Geometry: final body of the model. Coordinates: model frame, mm. A direction names the side the tool comes from. Round coordinates to 2 decimals unless told otherwise and drop trailing zeros. Loops run counter-clockwise (first coordinate to the right, second up) from the corner with the lowest first, then second, coordinate; pieces in that order, holes last. Notation, with made-up numbers: (-15.5, 80) - (21.5, 80) arc R21 ccw to (21.5, 93) - close; hole circle Ø5 at (-27, 3.5). An arc over 180 degrees is marked (long way). Use CSV: the item, a comma, the result in double quotes.
from build123d import *


with BuildPart() as f1:
    # F0 (on Front) → F1 (revolve)
    with BuildSketch(Plane.XZ):
        with BuildLine():
            Line((0, 49.5), (0, 0))
            Line((0, 0), (0, -47.5))
            Line((0, -47.5), (3.5, -52.52894))
            Line((3.5, -52.52894), (3.5, -56.52894))
            Line((3.5, -56.52894), (5.5, -56.52894))
            ThreePointArc((5.5, -56.52894), (6.132503, -53.02894), (5.5, -49.52894))
            ThreePointArc((5.5, -49.52894), (3.817857, -43.112045), (3, -36.52894))
            Line((3, -36.52894), (3, 0))
            Line((3, 0), (3, 34.5))
            ThreePointArc((3, 34.5), (3.570664, 41.066052), (5, 47.5))
            ThreePointArc((5, 47.5), (5.632503, 51), (5, 54.5))
            Line((5, 54.5), (3, 54.5))
            Line((3, 54.5), (3, 52.5))
            Line((3, 52.5), (0, 49.5))
        make_face()
    revolve(axis=Axis((-20.5, 0, 1.066906), (0, 0, -1)))


solid = f1.part
Item 1: Section B-B on y = 0. Return the cut outline in (x, z), plus the area to 3 significant figures.
Final values:
outline,"(-46.5, -56.53) - (-44.5, -56.53) - (-44.5, -52.53) - (-41, -47.5) - (-41, 49.5) - (-44, 52.5) - (-44, 54.5) - (-46, 54.5) arc R10 ccw to (-46, 47.5) arc R50 cw to (-44, 34.5) - (-44, -36.53) arc R50 cw to (-46.5, -49.53) arc R10 ccw to start; (0, -47.5) - (3.5, -52.53) - (3.5, -56.53) - (5.5, -56.53) arc R10 ccw to (5.5, -49.53) arc R50 cw to (3, -36.53) - (3, 34.5) arc R50 cw to (5, 47.5) arc R10 ccw to (5, 54.5) - (3, 54.5) - (3, 52.5) - (0, 49.5) - close"
area,"718 mm²"
Item 2: Mould query, pull axis X, two halves, no side actions, for faces 3 (the flat face through (-9, 21, 54.5)), 4 (the cylindrical face through (-39.55, 14.6, -54.56)), 5 (the cylindrical face through (-43.977, -1.033, -0.517)). Classes: released by +X, released by -X, zero draft, split by the parting line, or undercut.
Final values:
face 3,"zero draft"
face 4,"undercut"
face 5,"split by the parting line"
Item 3: Section A-A on x = -20.5. Return the cut outline in (y, z).
Final values:
outline,"(-26, -56.53) - (-24, -56.53) - (-24, -52.53) - (-20.5, -47.5) - (-20.5, 49.5) - (-23.5, 52.5) - (-23.5, 54.5) - (-25.5, 54.5) arc R10 ccw to (-25.5, 47.5) arc R50 cw to (-23.5, 34.5) - (-23.5, -36.53) arc R50 cw to (-26, -49.53) arc R10 ccw to start; (20.5, -47.5) - (24, -52.53) - (24, -56.53) - (26, -56.53) arc R10 ccw to (26, -49.53) arc R50 cw to (23.5, -36.53) - (23.5, 34.5) arc R50 cw to (25.5, 47.5) arc R10 ccw to (25.5, 54.5) - (23.5, 54.5) - (23.5, 52.5) - (20.5, 49.5) - close"
Item 4: Material intervals for line 1 (Y direction, x = -20.5, z = 28); line 2 (X direction, y = -0.5, z = -35); line 3 (Y direction, x = -24, z = -14), sorted ascending.
Final values:
line 1,"y = -23.5 to -20.5, 20.5 to 23.5"
line 2,"x = -43.99 to -40.99, -0.01 to 2.99"
line 3,"y = -23.24 to -20.2, 20.2 to 23.24"
Item 5: Pin query (flat end, axial travel): P1, Ø24.5, axis at x = -20.5, y = 0, coming from the +Z side; P2, Ø8, axis at x = -34, y = -11.5, coming from the -Z side; P3, Ø6, axis at y = -11.5, z = -8.5, coming from the -X side; P4, Ø3, axis at y = -15, z = -44, coming from the +X side. Return the tip coordinate at first contact, or that it passes through.
Final values:
P1,"passes through"
P2,"stops at z = -49.27"
P3,"stops at x = -42.41"
P4,"stops at x = 0.02"
Item 6: Reachability of faces 1 (the cylindrical face through (-37.82, -15.88, 53.49)), 2 (the cylindrical face through (-40.98, -0.9, 0.32)) from +Z, -Z, +X, -X, +Y, -Y: full face, straight path, thin tool, end or side. Return the list, or none.
Final values:
face 1,"+Z"
face 2,"+Z, -Z"
Item 7: Section D-D on z = -46. Return the cut outline in (x, y).
Final values:
outline,"circle Ø49.92 at (-20.5, 0); hole circle Ø41 at (-20.5, 0)"
Item 8: Section C-C on z = 21.5. Return the cut outline in (x, y).
Final values:
outline,"circle Ø47 at (-20.5, 0); hole circle Ø41 at (-20.5, 0)"
